Check sheet for the drawn part. Datum: minimum x, y, z corner. Units: mm. A direction names the side the tool comes from. Give positions to 0.01 mm unless a question says otherwise; leave off trailing zeros. Write each loop counter-clockwise with the first axis right and the second up, starting at its lowest first coordinate (ties: lowest second). Pieces come first, ordered by that corner, then holes. Notation, with made-up numbers: (2, 24.5) - (18, 24.5) arc R15 ccw to (18, 38.5) - close; hole circle Ø8 at (55, -24). An arc over 180 degrees is marked (long way). Return JSON: item names as keys, results as strings. Group by question number.
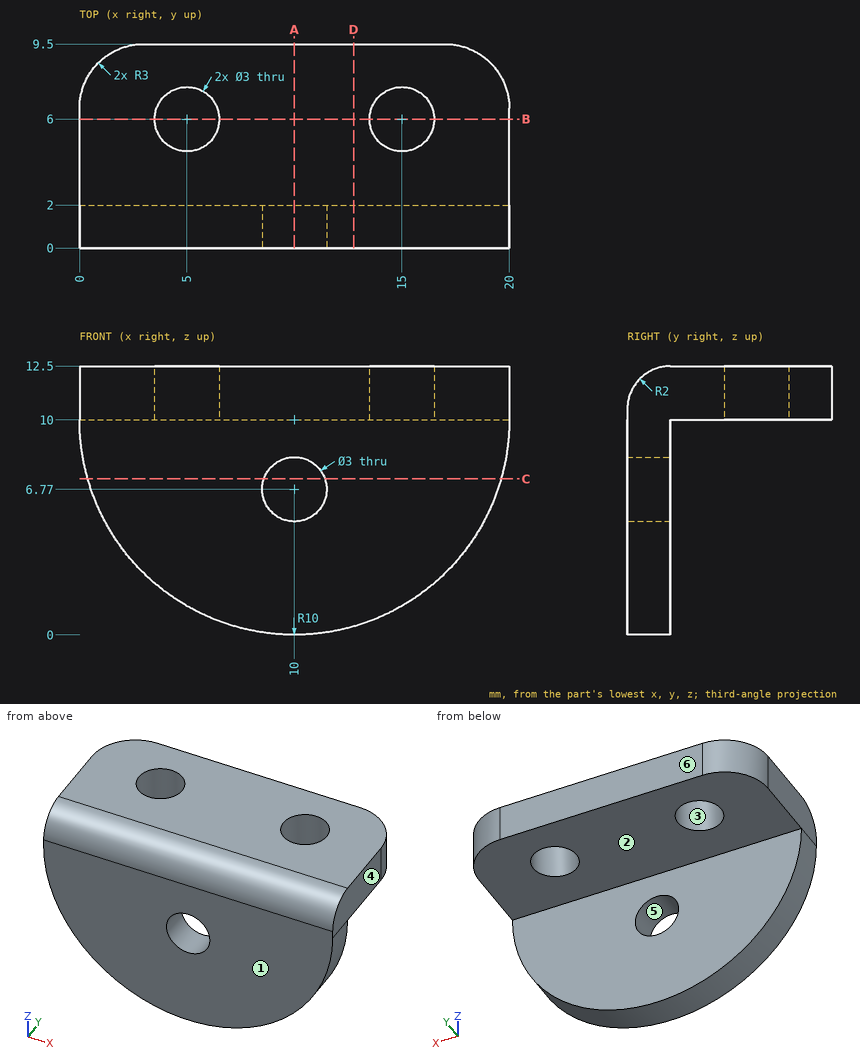
Item 1: Material ranges on line 1 along Y through (x, z) = (3, 5.5); line 2 along Z through (x, y) = (14.25, 4.25); line 3 along Y through (x, z) = (16.25, 11.5), recorded low to high. Write a range as from..to.
Item 2: Section check C-C on z = 7.25. Record the cut outline in (x, y).
Item 3: Access from +Z, -Z, +X, -X, +Y, -Y to the whole of each face (thin tool, end or side, straight path). Record for the marked faces 1 and 2.
Item 4: Section check D-D on x = 12.75. Record the cut outline in (y, z), plus the area to 3 significant figures.
Item 5: Mould release check, pull along X, two halves, no side actions. Record for the marked faces 3, 4, 5 and 6: +X half, -X half, draft (parallel to the pull), parting line (faces both ways), or undercut.
Item 6: Depth check by flat-ended pin: pin 1 (5 mm diameter, centred on x = 6.5, z = 5, fed in from +Y); pin 2 (3 mm diameter, centred on y = 2.5, z = 3.5, fed in from +X). Enter the tip coordinate at first touch or a pass-through.
Item 7: Section check A-A on x = 10. Record the cut outline in (y, z).
Item 8: Section check B-B on y = 6. Record the cut outline in (x, z).
Reply:
{
 "1": {"line 1": "0..2", "line 2": "10..12.5", "line 3": "0.27..5.17, 6.83..9.5"},
 "2": {"outline": "(0.39, 0) - (8.58, 0) - (8.58, 2) - (0.39, 2) - close; (11.42, 0) - (19.61, 0) - (19.61, 2) - (11.42, 2) - close"},
 "3": {"face 1": "+Z, -Z, +X, -X, -Y", "face 2": "-Z, +X, -X, +Y"},
 "4": {"outline": "(0, 0.39) - (2, 0.39) - (2, 10) - (9.5, 10) - (9.5, 12.5) - (2, 12.5) arc R2 ccw to (0, 10.5) - close", "area": "42.1 mm²"},
 "5": {"face 3": "undercut", "face 4": "+X half", "face 5": "undercut", "face 6": "draft"},
 "6": {"pin 1": "y = 2", "pin 2": "x = 18.61"},
 "7": {"outline": "(0, 0) - (2, 0) - (2, 5.27) - (0, 5.27) - close; (0, 8.27) - (2, 8.27) - (2, 10) - (9.5, 10) - (9.5, 12.5) - (2, 12.5) arc R2 ccw to (0, 10.5) - close"},
 "8": {"outline": "(0, 10) - (3.5, 10) - (3.5, 12.5) - (0, 12.5) - close; (6.5, 10) - (13.5, 10) - (13.5, 12.5) - (6.5, 12.5) - close; (16.5, 10) - (20, 10) - (20, 12.5) - (16.5, 12.5) - close"}
}
